Autodesk Inventor part; units mm, degrees
ref_plane "YZ Plane" through (0, 0, 0) normal (1, 0, 0) x (0, 1, 0)
ref_plane "XZ Plane" through (0, 0, 0) normal (0, 1, 0) x (-1, 0, 0)
ref_plane "XY Plane" through (0, 0, 0) normal (0, 0, 1) x (1, 0, 0)
sketch "Sketch1" plane through (0, 0, 0) normal (0, 0, 1) x (1, 0, 0)
  line L0 (0, 2.8582) -> (0, -2.8582) construction
  line L1 (-5.7775, 0) -> (5.7775, 0) construction
  circle A0 centre (0, 0) radius 26.3
  circle A1 centre (0, 0) radius 40
  line L2 (-40, 0) -> (-35, 0)
  circle A2 centre (-35, 0) radius 2.5
  line L3 (40, 0) -> (35, 0)
  circle A3 centre (35, 0) radius 2.5
  dimension "d0" = 52.6
  dimension "d1" = 80
  dimension "d4" = 5
  dimension "d5" = 5
  dimension "d6" = 5
  dimension "d7" = 5
extrude "Extrusion1" add sketch "Sketch1" along normal blind 5 contours A2 | A1 | A3
sketch "Sketch4" plane through (0, 0, 0) normal (0, 0, -1) x (-1, 0, 0)
  line L0 (0, 0) -> (-42, 0)
  line L1 (-42, 0) -> (42, 0)
  circle A0 centre (-42, 0) radius 2.5
  circle A1 centre (-42, 0) radius 6
  circle A2 centre (42, 0) radius 2.5
  circle A3 centre (42, 0) radius 6
  dimension "d19" = 42
  dimension "d20" = 84
  dimension "d21" = 5
  dimension "d22" = 12
  dimension "d23" = 5
  dimension "d24" = 12
extrude "Extrusion5" add sketch "Sketch4" against normal blind 5 contours A0 | A1 | A2 | A3
fillet "Fillet2" radius 12 4 edges at (39.619, -5.5074, 2.5) (39.619, 5.5074, 2.5) (-39.619, -5.5074, 2.5) (-39.619, 5.5074, 2.5)
extrude "Extrusion6" cut sketch "Sketch4" against normal blind 5 contours A0 | A2
sketch "Sketch5" plane through (0, 0, 5) normal (0, 0, 1) x (1, 0, 0)
  arc A0 (0, 29.3) -> (0, -29.3) centre (0, 0) ccw
  arc A1 (0, 31.3) -> (-4.25, -31.0101) centre (0, 0) ccw
  line L0 (0, 31.3) -> (0, 29.3)
  line L1 (0, -29.3) -> (4.25, -29.3)
  line L2 (4.25, -29.3) -> (4.25, -32.8)
  line L3 (4.25, -32.8) -> (-4.25, -32.8)
  line L4 (-4.25, -32.8) -> (-4.25, -31.0101)
  dimension "d30" = 29.3
  dimension "d31" = 31.3
  dimension "d32" = 4.25
  dimension "d33" = 3.5
  dimension "d34" = 8.5
extrude "Extrusion7" cut sketch "Sketch5" against normal blind 10
properties part number "Tussenplaat bevestiging axiale lager" material "S235"
Verification items for the finished model (mm, model axes). A direction names the side the tool comes from. Coordinates: 2 decimals unless noted, no trailing zeros. Write each loop counter-clockwise with the first axis right and the second up, starting at its lowest first coordinate (ties: lowest second). Pieces come first, ordered by that corner, then holes. Notation, with made-up numbers: M 27,86 L 47,86 A26 cw 47,124 Z; hole C 40,85 d9. An arc over 180 degrees is marked long. Use a Markdown table: item, result.
Q1. Sectioned sample at A-A, the plane y = 15. Record the boundary of the cut face in (x, z).
Reply:
| item | result |
|---|---|
| outline | M -37.08,0 L -27.47,0 L -27.47,5 L -37.08,5 Z; M -25.17,0 L -21.6,0 L -21.6,5 L -25.17,5 Z; M 21.6,0 L 37.08,0 L 37.08,5 L 21.6,5 Z |
Q2. Sectioned sample at D-D, the plane x = 27.5. Record the boundary of the cut face in (y, z).
Reply:
| item | result |
|---|---|
| outline | M -29.05,0 L 29.05,0 L 29.05,5 L -29.05,5 Z |
Q3. Sectioned sample at C-C, the plane z = 1.9. Count the separate pieces of the cut face and the enclosed holes in it, plus the area to 3 significant figures.
Reply:
| item | result |
|---|---|
| separate pieces | 1 |
| enclosed holes | 4 |
| area | 2,800 mm² |
Q4. Draft check along X on faces 1 (the face through (-29.293, 0.644, 2.535)), 2 (the face through (25, 12, 0)), 3 (the face through (0.699, -39.994, 2.465)). Enter one of: +X half, -X half, draft (parallel to the pull), parting line (faces both ways), or undercut.
Reply:
| item | result |
|---|---|
| face 1 | undercut |
| face 2 | draft |
| face 3 | parting line |
Q5. Sectioned sample at B-B, the plane x = 3. Record the boundary of the cut face in (y, z).
Reply:
| item | result |
|---|---|
| outline | M -39.89,0 L -32.8,0 L -32.8,5 L -39.89,5 Z; M -29.3,0 L -26.13,0 L -26.13,5 L -29.3,5 Z; M 26.13,0 L 39.89,0 L 39.89,5 L 26.13,5 Z |
Q6. Set-up check for faces 4 (the face through (4.25, -31, 3)), 5 (the face through (-48, 0, 2)): record each of +Z, -Z, +X, -X, +Y, -Y from which the full face is reachable in a straight line by a thin tool's end or side.
Reply:
| item | result |
|---|---|
| face 4 | +Z, -Z |
| face 5 | +Z, -Z, -X |
Q7. Thickness scan on line 1 (X direction, y = -5.5, z = 3.55); line 2 (X direction, y = 14.5, z = 4.75); line 3 (X direction, y = 1, z = 2.4). Record the ranges inside material, lowest first.
Reply:
| item | result |
|---|---|
| line 1 | x = -44.4 to -30.81, -28.78 to -25.72, 25.72 to 44.4 |
| line 2 | x = -37.28 to -27.74, -25.46 to -21.94, 21.94 to 37.28 |
| line 3 | x = -47.92 to -44.29, -39.71 to -31.28, -29.28 to -26.28, 26.28 to 39.71, 44.29 to 47.92 |
Q8. Go/stop test with flat-tipped pins: P1, Ø1.6, axis at y = 30.5, z = 1.5, coming from the -X side; P2, Ø1.4, axis at y = -32, z = 1.5, coming from the +X side; P3, Ø2.5, axis at x = 1.5, z = 2.5, coming from the +Y side. Record where each tip stops, or that it passes through.
Reply:
| item | result |
|---|---|
| P1 | stops at x = -26.79 |
| P2 | stops at x = 24.91 |
| P3 | stops at y = 40 |
